Print and shaded views of the part. All mm, measured from the part's lowest x, y and z. A direction names the side the tool comes from. Round coordinates to 2 decimals unless told otherwise and drop trailing zeros. Write each loop counter-clockwise with the first axis right and the second up, starting at its lowest first coordinate (ties: lowest second). Pieces come first, ordered by that corner, then holes. Notation, with made-up numbers: (23.25, 51.5) - (39.25, 51.5) arc R20 cw to (39.25, 55.5) - close; hole circle Ø4 at (24, 57.25). An arc over 180 degrees is marked (long way). Put each result on its own line as item: value. Start each with the question number.
Item 1: Cut at B-B (z = 56.5). Give the cut face in (x, y).
Item 2: Cut at A-A (y = 134). Give the cut face in (x, z), and give its area (3 significant figures).
Item 3: Drill centre lines: line 1 (X direction, y = 102, z = 37) (1 decimal); line 2 (X direction, y = 121.5, z = 67) (1 decimal); line 3 (Z direction, x = 63, y = 135) (1 decimal). Where is each one in solid material? Low to high. Write a range as from..to.
Item 4: Cut at D-D (z = 35). Give the cut face in (x, y).
Item 5: 3-axis set-ups, long thin cutter, end or side, ignore diameter. For the marked faces 1 and 2: which of +Z, -Z, +X, -X, +Y, -Y reach the whole face in a straight line?
Item 6: Mould opens along X. For the marked faces 3, 4 and 5 say: released by +X, released by -X, zero draft, split by the parting line, or undercut.
Item 7: Pin check, flat tips, straight feed: pin 1 Ø12 at (y, z) = (42, 20) entering from -X; pin 2 Ø1.5 at (x, y) = (40.5, 108.5) entering from -Z. Stop position of each tip, or through.
Item 8: Cut at C-C (x = 18). Give the cut face in (y, z), and give its area (3 significant figures).
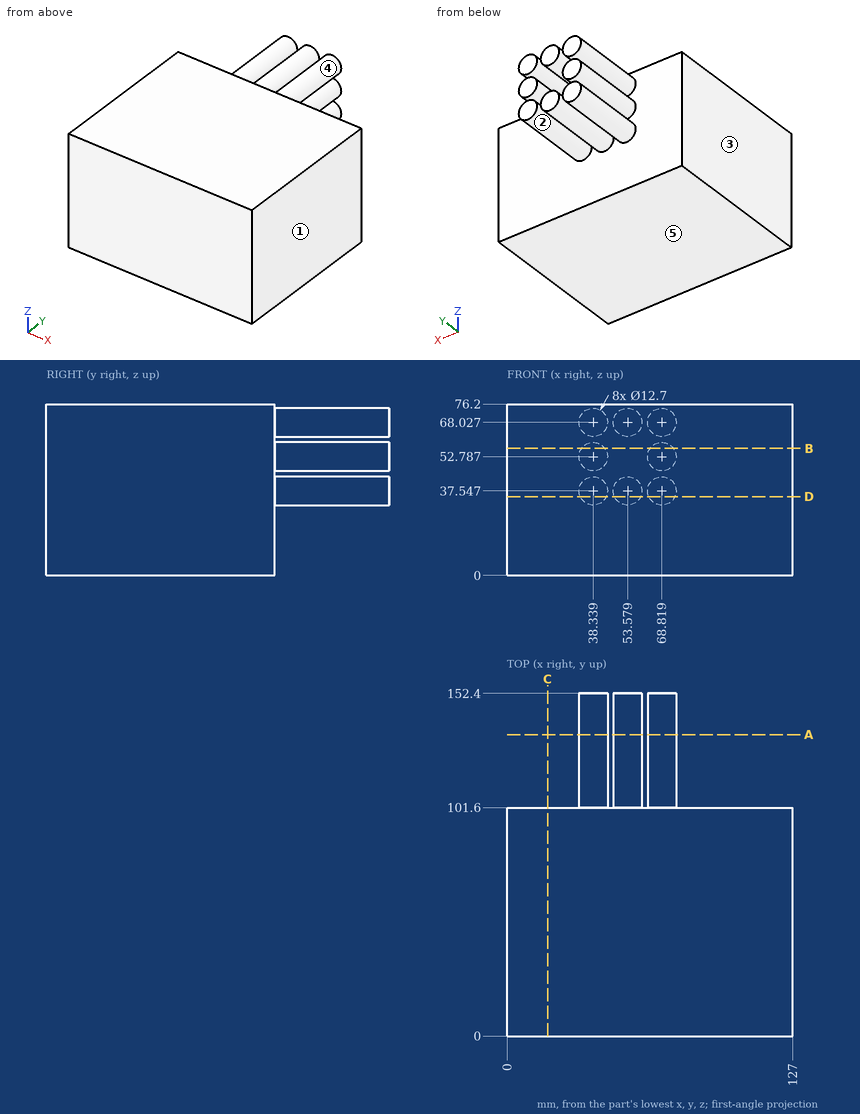
Output values:
1. outline: (0, 0) - (127, 0) - (127, 101.6) - (73.97, 101.6) - (73.97, 152.4) - (63.67, 152.4) - (63.67, 101.6) - (43.49, 101.6) - (43.49, 152.4) - (33.19, 152.4) - (33.19, 101.6) - (0, 101.6) - close
2. outline: circle Ø12.7 at (38.34, 37.55); circle Ø12.7 at (38.34, 52.79); circle Ø12.7 at (38.34, 68.03); circle Ø12.7 at (53.58, 37.55); circle Ø12.7 at (53.58, 68.03); circle Ø12.7 at (68.82, 37.55); circle Ø12.7 at (68.82, 52.79); circle Ø12.7 at (68.82, 68.03)
2. area: 1,010 mm2
3. line 1: 32..44.7, 47.3..59.9, 62.5..75.1
3. line 2: 32.1..44.6, 47.3..59.8, 62.6..75.1
3. line 3: 35..40.1, 50.2..55.3, 65.5..70.6
4. outline: (0, 0) - (127, 0) - (127, 101.6) - (74.64, 101.6) - (74.64, 152.4) - (63, 152.4) - (63, 101.6) - (59.4, 101.6) - (59.4, 152.4) - (47.76, 152.4) - (47.76, 101.6) - (44.16, 101.6) - (44.16, 152.4) - (32.52, 152.4) - (32.52, 101.6) - (0, 101.6) - close
5. face 1: +Z, -Z, +X, +Y, -Y
5. face 2: +Y
6. face 3: released by -X
6. face 4: undercut
6. face 5: zero draft
7. pin 1: x = 0
7. pin 2: z = 31.36
8. outline: (0, 0) - (101.6, 0) - (101.6, 76.2) - (0, 76.2) - close
8. area: 7,740 mm2
